Build history of the part. All positions in model axes, mm. A direction names the side the tool comes from. Round coordinates to 2 decimals unless told otherwise and drop trailing zeros. Write each loop counter-clockwise with the first axis right and the second up, starting at its lowest first coordinate (ties: lowest second). Pieces come first, ordered by that corner, then holes.
Autodesk Inventor part; units mm, degrees
ref_plane "開始平面" through (0, 0, 0) normal (0, 1, 0) x (-1, 0, 0)
ref_plane "終了平面" through (0, 196, 0) normal (0, 1, 0) x (-1, 0, 0)
ref_plane "YZ Plane" through (0, 0, 0) normal (1, 0, 0) x (0, 1, 0)
ref_plane "開始平面" through (0, 0, 0) normal (0, 1, 0) x (-1, 0, 0)
ref_plane "終了平面" through (0, 196, 0) normal (0, 1, 0) x (-1, 0, 0)
sketch "スケッチ" plane through (0, 0, 0) normal (0, 1, 0) x (-1, 0, 0)
  line L0 (8.5, -3.8) -> (8.5, -2.6)
  line L1 (4, -8.3) -> (4, -5)
  circle A0 centre (7, -7) radius 2
  line L2 (10, -2.6) -> (10, -9.5)
  line L3 (2.6, -10) -> (9.5, -10)
  line L4 (2.1, -9.5) -> (2.1, -9)
  line L5 (8.5, -2.1) -> (8.5, -4)
  line L6 (3.8, -4.8) -> (2.6, -4.8)
  line L7 (4.8, -3.8) -> (4.8, -2.6)
  arc A1 (2.1, -4.3) -> (2.6, -4.8) centre (2.6, -4.3) ccw
  arc A2 (2.6, -8.5) -> (2.1, -9) centre (2.6, -9) ccw
  arc A3 (3.8, -8.5) -> (4, -8.3) centre (3.8, -8.3) ccw
  arc A4 (4, -5) -> (3.8, -4.8) centre (3.8, -5) ccw
  arc A5 (2.1, -3.5) -> (1.6, -3) centre (1.6, -3.5) ccw
  arc A6 (2.1, -9.5) -> (2.6, -10) centre (2.6, -9.5) ccw
  arc A7 (9.5, -10) -> (10, -9.5) centre (9.5, -9.5) ccw
  arc A8 (10, -2.6) -> (9.5, -2.1) centre (9.5, -2.6) ccw
  arc A9 (9, -2.1) -> (8.5, -2.6) centre (9, -2.6) ccw
  arc A10 (8.3, -4) -> (8.5, -3.8) centre (8.3, -3.8) ccw
  arc A11 (4.8, -3.8) -> (5, -4) centre (5, -3.8) ccw
  line L8 (4.3, -2.1) -> (3.5, -2.1)
  arc A12 (4.8, -2.6) -> (4.3, -2.1) centre (4.3, -2.6) ccw
  arc A13 (3, -1.6) -> (3.5, -2.1) centre (3.5, -1.6) ccw
  line L9 (2.1, -4.3) -> (2.1, -3.5)
  line L10 (3.8, -8.5) -> (2.6, -8.5)
  line L11 (9.5, -2.1) -> (9, -2.1)
  line L12 (8.3, -4) -> (5, -4)
  circle A14 centre (0, 0) radius 1.65
  arc A15 (8.5, 2.6) -> (9, 2.1) centre (9, 2.6) ccw
  line L13 (8.5, 3.8) -> (8.5, 2.6)
  arc A16 (8.5, 3.8) -> (8.3, 4) centre (8.3, 3.8) ccw
  line L14 (8.3, 4) -> (5, 4)
  line L15 (10, 2.6) -> (10, 9.5)
  arc A17 (10, 9.5) -> (9.5, 10) centre (9.5, 9.5) ccw
  circle A18 centre (7, 7) radius 2
  line L16 (4, 8.3) -> (4, 5)
  line L17 (2.6, 10) -> (9.5, 10)
  line L18 (9.5, 2.1) -> (9, 2.1)
  arc A19 (9.5, 2.1) -> (10, 2.6) centre (9.5, 2.6) ccw
  line L19 (3.8, 8.5) -> (2.6, 8.5)
  line L20 (4.8, 3.8) -> (4.8, 2.6)
  arc A20 (4.3, 2.1) -> (4.8, 2.6) centre (4.3, 2.6) ccw
  line L21 (2.1, 8.5) -> (4, 8.5)
  arc A21 (4, 8.3) -> (3.8, 8.5) centre (3.8, 8.3) ccw
  arc A22 (2.1, 9) -> (2.6, 8.5) centre (2.6, 9) ccw
  arc A23 (2.6, 10) -> (2.1, 9.5) centre (2.6, 9.5) ccw
  line L22 (2.1, 9.5) -> (2.1, 9)
  arc A24 (1.6, 3) -> (2.1, 3.5) centre (1.6, 3.5) ccw
  line L23 (3.8, 4.8) -> (2.6, 4.8)
  arc A25 (5, 4) -> (4.8, 3.8) centre (5, 3.8) ccw
  arc A26 (3.8, 4.8) -> (4, 5) centre (3.8, 5) ccw
  line L24 (4.3, 2.1) -> (3.5, 2.1)
  arc A27 (2.6, 4.8) -> (2.1, 4.3) centre (2.6, 4.3) ccw
  line L25 (2.1, 4.3) -> (2.1, 3.5)
  arc A28 (3.5, 2.1) -> (3, 1.6) centre (3.5, 1.6) ccw
  arc A29 (-2.6, 8.5) -> (-2.1, 9) centre (-2.6, 9) ccw
  line L26 (-3.8, 8.5) -> (-2.6, 8.5)
  arc A30 (-3.8, 8.5) -> (-4, 8.3) centre (-3.8, 8.3) ccw
  line L27 (-4, 8.3) -> (-4, 5)
  line L28 (-2.6, 10) -> (-9.5, 10)
  arc A31 (-9.5, 10) -> (-10, 9.5) centre (-9.5, 9.5) ccw
  circle A32 centre (-7, 7) radius 2
  line L29 (-8.3, 4) -> (-5, 4)
  line L30 (-10, 2.6) -> (-10, 9.5)
  line L31 (-2.1, 9.5) -> (-2.1, 9)
  arc A33 (-2.1, 9.5) -> (-2.6, 10) centre (-2.6, 9.5) ccw
  line L32 (-8.5, 3.8) -> (-8.5, 2.6)
  line L33 (-3.8, 4.8) -> (-2.6, 4.8)
  arc A34 (-2.1, 4.3) -> (-2.6, 4.8) centre (-2.6, 4.3) ccw
  line L34 (-8.5, 2.1) -> (-8.5, 4)
  arc A35 (-8.3, 4) -> (-8.5, 3.8) centre (-8.3, 3.8) ccw
  arc A36 (-9, 2.1) -> (-8.5, 2.6) centre (-9, 2.6) ccw
  arc A37 (-10, 2.6) -> (-9.5, 2.1) centre (-9.5, 2.6) ccw
  line L35 (-9.5, 2.1) -> (-9, 2.1)
  arc A38 (-3, 1.6) -> (-3.5, 2.1) centre (-3.5, 1.6) ccw
  line L36 (-4.8, 3.8) -> (-4.8, 2.6)
  arc A39 (-4, 5) -> (-3.8, 4.8) centre (-3.8, 5) ccw
  arc A40 (-4.8, 3.8) -> (-5, 4) centre (-5, 3.8) ccw
  line L37 (-2.1, 4.3) -> (-2.1, 3.5)
  arc A41 (-4.8, 2.6) -> (-4.3, 2.1) centre (-4.3, 2.6) ccw
  line L38 (-4.3, 2.1) -> (-3.5, 2.1)
  arc A42 (-2.1, 3.5) -> (-1.6, 3) centre (-1.6, 3.5) ccw
  arc A43 (-8.5, -2.6) -> (-9, -2.1) centre (-9, -2.6) ccw
  line L39 (-8.5, -3.8) -> (-8.5, -2.6)
  arc A44 (-8.5, -3.8) -> (-8.3, -4) centre (-8.3, -3.8) ccw
  line L40 (-8.3, -4) -> (-5, -4)
  line L41 (-10, -2.6) -> (-10, -9.5)
  arc A45 (-10, -9.5) -> (-9.5, -10) centre (-9.5, -9.5) ccw
  circle A46 centre (-7, -7) radius 2
  line L42 (-4, -8.3) -> (-4, -5)
  line L43 (-2.6, -10) -> (-9.5, -10)
  line L44 (-9.5, -2.1) -> (-9, -2.1)
  arc A47 (-9.5, -2.1) -> (-10, -2.6) centre (-9.5, -2.6) ccw
  line L45 (-3.8, -8.5) -> (-2.6, -8.5)
  line L46 (-4.8, -3.8) -> (-4.8, -2.6)
  arc A48 (-4.3, -2.1) -> (-4.8, -2.6) centre (-4.3, -2.6) ccw
  line L47 (-2.1, -8.5) -> (-4, -8.5)
  arc A49 (-4, -8.3) -> (-3.8, -8.5) centre (-3.8, -8.3) ccw
  arc A50 (-2.1, -9) -> (-2.6, -8.5) centre (-2.6, -9) ccw
  arc A51 (-2.6, -10) -> (-2.1, -9.5) centre (-2.6, -9.5) ccw
  line L48 (-2.1, -9.5) -> (-2.1, -9)
  arc A52 (-1.6, -3) -> (-2.1, -3.5) centre (-1.6, -3.5) ccw
  line L49 (-3.8, -4.8) -> (-2.6, -4.8)
  arc A53 (-5, -4) -> (-4.8, -3.8) centre (-5, -3.8) ccw
  arc A54 (-3.8, -4.8) -> (-4, -5) centre (-3.8, -5) ccw
  line L50 (-4.3, -2.1) -> (-3.5, -2.1)
  arc A55 (-2.6, -4.8) -> (-2.1, -4.3) centre (-2.6, -4.3) ccw
  line L51 (-2.1, -4.3) -> (-2.1, -3.5)
  arc A56 (-3.5, -2.1) -> (-3, -1.6) centre (-3.5, -1.6) ccw
  line L52 (1.6, -3) -> (-1.6, -3)
  line L53 (-3, -1.6) -> (-3, 1.6)
  line L54 (-1.6, 3) -> (1.6, 3)
  line L55 (3, 1.6) -> (3, -1.6)
  point P0 (2.1, -10)
  point P1 (10, 2.1)
  point P2 (-2.1, 10)
  point P3 (-10, -2.1)
  dimension "d12" = 4
  dimension "d14" = 3.7
  dimension "d16" = 0.5
  dimension "d17" = 0.5
  dimension "d18" = 0.2
  dimension "d19" = 0.5
  dimension "d20" = 0.5
  dimension "d24" = 0.5
  dimension "d25" = 0.2
  dimension "d28" = 0.5
  dimension "d31" = 1.5
  dimension "d36" = 3.7
  dimension "d37" = 1.5
  dimension "d58" = 3.3
  dimension "d65" = 10
  dimension "d67" = 2.1
  dimension "d68" = 2.1
  dimension "d69" = 1.9
  dimension "d70" = 7
  dimension "d72" = 2.1
  dimension "d73" = 2.1
  dimension "d74" = 1.9
  dimension "d75" = 7
  dimension "d76" = 10
  dimension "d80" = 360
  dimension "d82" = 3
extrude "ボディ" add sketch "スケッチ" along normal up to surface (196 mm away) from surface at 0
sketch "スケッチ4" plane through (0, 0, 0) normal (0, 1, 0) x (-1, 0, 0)
  line L0 (0, 0) -> (10, 0)
ref_plane "作業平面4" through (0, 0, 0) normal (0, 0, -1) x (-1, 0, 0)
sketch "スケッチ5" plane through (0, 0, 0) normal (0, 0, -1) x (-1, 0, 0)
  line L0 (-2, 0) -> (12, 0)
  line L1 (-2, 196) -> (12, 196)
sketch "スケッチ9" plane through (2.6, 0, -10) normal (0, -1, 0) x (1, 0, 0)
  circle A0 centre (4.4, 3) radius 2
  circle A1 centre (4.4, 17) radius 2
  circle A2 centre (-9.6, 17) radius 2
  circle A3 centre (-9.6, 3) radius 2
  circle A4 centre (-2.6, 10) radius 1.65
  arc A5 (-5.2, 5.2) -> (-4.7, 5.7) centre (-5.2, 5.7) ccw
  line L0 (-4.7, 5.7) -> (-4.7, 6.5)
  arc A6 (-4.2, 7) -> (-4.7, 6.5) centre (-4.2, 6.5) ccw
  line L1 (-4.2, 7) -> (-1, 7)
  arc A7 (-0.5, 6.5) -> (-1, 7) centre (-1, 6.5) ccw
  line L2 (-0.5, 6.5) -> (-0.5, 5.7)
  arc A8 (-0.5, 5.7) -> (0, 5.2) centre (0, 5.7) ccw
  line L3 (0, 5.2) -> (1.2, 5.2)
  arc A9 (1.4, 5) -> (1.2, 5.2) centre (1.2, 5) ccw
  line L4 (1.4, 5) -> (1.4, 1.7)
  arc A10 (1.2, 1.5) -> (1.4, 1.7) centre (1.2, 1.7) ccw
  line L5 (1.2, 1.5) -> (0, 1.5)
  arc A11 (0, 1.5) -> (-0.5, 1) centre (0, 1) ccw
  line L6 (-0.5, 1) -> (-0.5, 0.5)
  arc A12 (-0.5, 0.5) -> (0, 0) centre (0, 0.5) ccw
  line L7 (0, 0) -> (6.9, 0)
  arc A13 (6.9, 0) -> (7.4, 0.5) centre (6.9, 0.5) ccw
  line L8 (7.4, 0.5) -> (7.4, 7.4)
  arc A14 (7.4, 7.4) -> (6.9, 7.9) centre (6.9, 7.4) ccw
  line L9 (6.9, 7.9) -> (6.4, 7.9)
  arc A15 (6.4, 7.9) -> (5.9, 7.4) centre (6.4, 7.4) ccw
  line L10 (5.9, 7.4) -> (5.9, 6.2)
  arc A16 (5.7, 6) -> (5.9, 6.2) centre (5.7, 6.2) ccw
  line L11 (5.7, 6) -> (2.4, 6)
  arc A17 (2.2, 6.2) -> (2.4, 6) centre (2.4, 6.2) ccw
  line L12 (2.2, 6.2) -> (2.2, 7.4)
  arc A18 (2.2, 7.4) -> (1.7, 7.9) centre (1.7, 7.4) ccw
  line L13 (1.7, 7.9) -> (0.9, 7.9)
  arc A19 (0.4, 8.4) -> (0.9, 7.9) centre (0.9, 8.4) ccw
  line L14 (0.4, 8.4) -> (0.4, 11.6)
  arc A20 (0.9, 12.1) -> (0.4, 11.6) centre (0.9, 11.6) ccw
  line L15 (0.9, 12.1) -> (1.7, 12.1)
  arc A21 (1.7, 12.1) -> (2.2, 12.6) centre (1.7, 12.6) ccw
  line L16 (2.2, 12.6) -> (2.2, 13.8)
  arc A22 (2.4, 14) -> (2.2, 13.8) centre (2.4, 13.8) ccw
  line L17 (2.4, 14) -> (5.7, 14)
  arc A23 (5.9, 13.8) -> (5.7, 14) centre (5.7, 13.8) ccw
  line L18 (5.9, 13.8) -> (5.9, 12.6)
  arc A24 (5.9, 12.6) -> (6.4, 12.1) centre (6.4, 12.6) ccw
  line L19 (6.4, 12.1) -> (6.9, 12.1)
  arc A25 (6.9, 12.1) -> (7.4, 12.6) centre (6.9, 12.6) ccw
  line L20 (7.4, 12.6) -> (7.4, 19.5)
  arc A26 (7.4, 19.5) -> (6.9, 20) centre (6.9, 19.5) ccw
  line L21 (6.9, 20) -> (0, 20)
  arc A27 (0, 20) -> (-0.5, 19.5) centre (0, 19.5) ccw
  line L22 (-0.5, 19.5) -> (-0.5, 19)
  arc A28 (-0.5, 19) -> (0, 18.5) centre (0, 19) ccw
  line L23 (0, 18.5) -> (1.2, 18.5)
  arc A29 (1.4, 18.3) -> (1.2, 18.5) centre (1.2, 18.3) ccw
  line L24 (1.4, 18.3) -> (1.4, 15)
  arc A30 (1.2, 14.8) -> (1.4, 15) centre (1.2, 15) ccw
  line L25 (1.2, 14.8) -> (0, 14.8)
  arc A31 (0, 14.8) -> (-0.5, 14.3) centre (0, 14.3) ccw
  line L26 (-0.5, 14.3) -> (-0.5, 13.5)
  arc A32 (-1, 13) -> (-0.5, 13.5) centre (-1, 13.5) ccw
  line L27 (-1, 13) -> (-4.2, 13)
  arc A33 (-4.7, 13.5) -> (-4.2, 13) centre (-4.2, 13.5) ccw
  line L28 (-4.7, 13.5) -> (-4.7, 14.3)
  arc A34 (-4.7, 14.3) -> (-5.2, 14.8) centre (-5.2, 14.3) ccw
  line L29 (-5.2, 14.8) -> (-6.4, 14.8)
  arc A35 (-6.6, 15) -> (-6.4, 14.8) centre (-6.4, 15) ccw
  line L30 (-6.6, 15) -> (-6.6, 18.3)
  arc A36 (-6.4, 18.5) -> (-6.6, 18.3) centre (-6.4, 18.3) ccw
  line L31 (-6.4, 18.5) -> (-5.2, 18.5)
  arc A37 (-5.2, 18.5) -> (-4.7, 19) centre (-5.2, 19) ccw
  line L32 (-4.7, 19) -> (-4.7, 19.5)
  arc A38 (-4.7, 19.5) -> (-5.2, 20) centre (-5.2, 19.5) ccw
  line L33 (-5.2, 20) -> (-12.1, 20)
  arc A39 (-12.1, 20) -> (-12.6, 19.5) centre (-12.1, 19.5) ccw
  line L34 (-12.6, 19.5) -> (-12.6, 12.6)
  arc A40 (-12.6, 12.6) -> (-12.1, 12.1) centre (-12.1, 12.6) ccw
  line L35 (-12.1, 12.1) -> (-11.6, 12.1)
  arc A41 (-11.6, 12.1) -> (-11.1, 12.6) centre (-11.6, 12.6) ccw
  line L36 (-11.1, 12.6) -> (-11.1, 13.8)
  arc A42 (-10.9, 14) -> (-11.1, 13.8) centre (-10.9, 13.8) ccw
  line L37 (-10.9, 14) -> (-7.6, 14)
  arc A43 (-7.4, 13.8) -> (-7.6, 14) centre (-7.6, 13.8) ccw
  line L38 (-7.4, 13.8) -> (-7.4, 12.6)
  arc A44 (-7.4, 12.6) -> (-6.9, 12.1) centre (-6.9, 12.6) ccw
  line L39 (-6.9, 12.1) -> (-6.1, 12.1)
  arc A45 (-5.6, 11.6) -> (-6.1, 12.1) centre (-6.1, 11.6) ccw
  line L40 (-5.6, 11.6) -> (-5.6, 8.4)
  arc A46 (-6.1, 7.9) -> (-5.6, 8.4) centre (-6.1, 8.4) ccw
  line L41 (-6.1, 7.9) -> (-6.9, 7.9)
  arc A47 (-6.9, 7.9) -> (-7.4, 7.4) centre (-6.9, 7.4) ccw
  line L42 (-7.4, 7.4) -> (-7.4, 6.2)
  arc A48 (-7.6, 6) -> (-7.4, 6.2) centre (-7.6, 6.2) ccw
  line L43 (-7.6, 6) -> (-10.9, 6)
  arc A49 (-11.1, 6.2) -> (-10.9, 6) centre (-10.9, 6.2) ccw
  line L44 (-11.1, 6.2) -> (-11.1, 7.4)
  arc A50 (-11.1, 7.4) -> (-11.6, 7.9) centre (-11.6, 7.4) ccw
  line L45 (-11.6, 7.9) -> (-12.1, 7.9)
  arc A51 (-12.1, 7.9) -> (-12.6, 7.4) centre (-12.1, 7.4) ccw
  line L46 (-12.6, 7.4) -> (-12.6, 0.5)
  arc A52 (-12.6, 0.5) -> (-12.1, 0) centre (-12.1, 0.5) ccw
  line L47 (-12.1, 0) -> (-5.2, 0)
  arc A53 (-5.2, 0) -> (-4.7, 0.5) centre (-5.2, 0.5) ccw
  line L48 (-4.7, 0.5) -> (-4.7, 1)
  arc A54 (-4.7, 1) -> (-5.2, 1.5) centre (-5.2, 1) ccw
  line L49 (-5.2, 1.5) -> (-6.4, 1.5)
  arc A55 (-6.6, 1.7) -> (-6.4, 1.5) centre (-6.4, 1.7) ccw
  line L50 (-6.6, 1.7) -> (-6.6, 5)
  arc A56 (-6.4, 5.2) -> (-6.6, 5) centre (-6.4, 5) ccw
  line L51 (-6.4, 5.2) -> (-5.2, 5.2)
  line L52 (6.9, 20) -> (0, 20)
  line L53 (-5.2, 20) -> (0, 20)
  line L54 (7.4, 12.6) -> (7.4, 19.5)
  line L55 (7.4, 12.6) -> (7.4, 7.4)
extrude "押し出し7" add sketch "スケッチ9" against normal blind 196 contours A1 | A14 L9 A15 L10 A16 L11 A17 L12 A18 L13 A19 L14 A20 L15 A21 L16 A22 L17 A23 L18 A24 L19 A25 L55 | A27 L22 A28 L23 A29 L24 A30 L25 A31 L26 A32 L27 A33 L28 A34 L29 A35 L30 A36 L31 A37 L32 A38 L53
sketch "スケッチ10" plane through (-9.5, 0, 10) normal (0, -1, 0) x (1, 0, 0)
  line L0 (-0.5, -12.6) -> (-0.5, -19.5) construction
  line L1 (0, -20) -> (6.9, -20) construction
  arc A0 (-0.5, -19.5) -> (0, -20) centre (0, -19.5) ccw construction
  line L2 (-0.5, -19.5) -> (-0.5, -20) construction
  line L3 (-0.5, -20) -> (0, -20) construction
  arc A1 (0, 0) -> (-0.5, -0.5) centre (0, -0.5) ccw
  arc A2 (19.4953, -19.5681) -> (-0.0681, -0.0047) centre (-0.5, -20) ccw
  line L4 (19, 0) -> (0, 0)
  arc A3 (19.5, -0.5) -> (19, 0) centre (19, -0.5) ccw
  line L5 (19.5, -19.5) -> (19.5, -0.5)
  arc A4 (19, -20) -> (19.5, -19.5) centre (19, -19.5) ccw
  point P0 (9.5, -10)
  dimension "d101" = 20
extrude "押し出し8" cut sketch "スケッチ10" against normal through all
equation "\"d99\" = Length"
equation "\"Length\" = 196"
equation "\"G_OFFSET_START\" = 0"
equation "\"G_OFFSET_END\" = 0"
equation "\"d86\" = Length + G_OFFSET_END"
equation "\"G_L\" = 196"
properties part number "r150" material "アルミニウム 6061"
1) Mould opens along X. For faces 1 (the cylindrical face through (4.29, 96.63, 3.99)), 2 (the flat face through (-7, 97, -4)), 3 (the flat face through (-6, 97, -10)) say: released by +X, released by -X, zero draft, split by the parting line, or undercut.
Results:
face 1: released by +X
face 2: undercut
face 3: zero draft
2) Pin check, flat tips, straight feed: pin 1 Ø1 at (y, z) = (122.5, -8) entering from +X; pin 2 Ø6 at (x, y) = (7.5, 97) entering from +Z; pin 3 Ø3.5 at (x, y) = (-6, 51) entering from +Z. Stop position of each tip, or through.
Results:
pin 1: stops at x = 9.94
pin 2: stops at z = 3.77
pin 3: stops at z = 9.87
3) Slice it at A-A (z = 0). Write the cut outline in (x, y).
Results:
outline: (-3, 0) - (-1.65, 0) - (-1.65, 196) - (-3, 196) - close; (1.65, 0) - (7.32, 0) - (7.32, 196) - (1.65, 196) - close
4) Slice it at C-C (y = 156.5). Count the separate pieces of the cut face and the enclosed holes in it, plus the area to 3 significant figures.
Results:
separate pieces: 1
enclosed holes: 4
area: 180 mm2
5) Slice it at B-B (x = 0). Write the cut outline in (y, z).
Results:
outline: (0, -3) - (196, -3) - (196, -1.65) - (0, -1.65) - close; (0, 1.65) - (196, 1.65) - (196, 7.32) - (0, 7.32) - close
6) Which spindle directions (+Z, -Z, +X, -X, +Y, -Y) get a long thin tool onto all of the face, cutting with end or side? Do faces 4 (the flat face through (0, 196, -2)), 5 (the flat face through (-4, 97, -7)), 6 (the flat face through (-3, 97, 0)), 7 (the flat face through (0, 97, -3)). Say none if no direction does.
Results:
face 4: +Z, -Z, +X, -X, +Y
face 5: +Y, -Y
face 6: -X, +Y, -Y
face 7: -Z, +Y, -Y
7) Wall check: L1, parallel to Z at x = -3.75, y = 148; L2, parallel to X at y = 14, z = -6.5; L3, parallel to X at y = 59, z = -7.5. Give the ranges that are in metal, low to high.
Results:
L1: z = -10 to -8.5, -4.8 to -2.1, 2.1 to 9
L2: x = -10 to -8.94, -5.06 to -4, 4 to 5.06, 8.94 to 9.69
L3: x = -10 to -8.94, -5.06 to -4, 4 to 5.06, 8.94 to 9.84
